Work out the finished part from the listing and answer in its coordinate system (mm). Coordinates: 2 decimals unless noted, no trailing zeros. Order: outer loops, then holes, each group sorted by start corner. A loop starts at its lowest first (then second) coordinate and runs counter-clockwise, first axis right, second up. Notation, with made-up numbers: M -34.5,11.5 L 8.5,11.5 A32 cw 8.5,49.5 Z; hole C -8.75,4.5 d3. An arc over 180 degrees is marked long. Use a Markdown table: item, result.
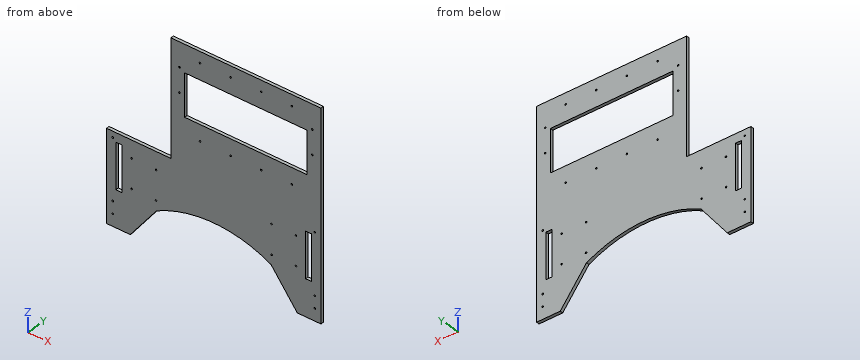
from build123d import *

# Parameters (mm, degrees)
SKETCH1_R           = 1.63195
SKETCH1_W           = 254
SKETCH1_H           = 88.9
SKETCH1_W_2         = 12.7
SKETCH1_H_2         = 95.25
BOSS_EXTRUDE1_DEPTH = 6.35
CUT_EXTRUDE1_REACH  = 621.735
SKETCH2_R           = 1.63195
CUT_EXTRUDE2_REACH  = 621.735
SKETCH4_R           = 1.63195


with BuildPart() as part:
    # Sketch1 → Boss-Extrude1 (new body)
    with BuildSketch(Plane(origin=(0, 0, 0), x_dir=(1, 0, 0), z_dir=(0, 1, 0))):
        with BuildLine():
            Line((-444.5, 431.8), (-395.456941666, 431.8))
            Line((-395.456941666, 431.8), (-340.943704665, 359.56166268))
            ThreePointArc((-340.943704665, 359.56166268), (-222.25, 330.203093028), (-103.556295335, 359.56166268))
            Line((-103.556295335, 359.56166268), (-49.043058334, 431.8))
            Line((-49.043058334, 431.8), (0, 431.8))
            Line((0, 431.8), (0, 0))
            Line((0, 0), (-311.15, 0))
            Line((-311.15, 0), (-311.15, 241.3))
            Line((-311.15, 241.3), (-444.5, 241.3))
            Line((-444.5, 241.3), (-444.5, 431.8))
        make_face()
        with Locations(Location((-250.825, 23.368, 0), (0, 0, 270))):
            Circle(SKETCH1_R, mode=Mode.SUBTRACT)
        with Locations(Location((-187.325, 23.368, 0), (0, 0, 270))):
            Circle(SKETCH1_R, mode=Mode.SUBTRACT)
        with Locations(Location((-187.325, 179.8955, 0), (0, 0, 270))):
            Circle(SKETCH1_R, mode=Mode.SUBTRACT)
        with Locations(Location((-250.825, 179.8955, 0), (0, 0, 270))):
            Circle(SKETCH1_R, mode=Mode.SUBTRACT)
        with Locations(Location((-123.825, 179.8955, 0), (0, 0, 270))):
            Circle(SKETCH1_R, mode=Mode.SUBTRACT)
        with Locations(Location((-60.325, 179.8955, 0), (0, 0, 270))):
            Circle(SKETCH1_R, mode=Mode.SUBTRACT)
        with Locations(Location((-123.825, 23.368, 0), (0, 0, 270))):
            Circle(SKETCH1_R, mode=Mode.SUBTRACT)
        with Locations(Location((-60.325, 23.368, 0), (0, 0, 270))):
            Circle(SKETCH1_R, mode=Mode.SUBTRACT)
        with Locations((-155.575, 101.63175)):
            Rectangle(SKETCH1_W, SKETCH1_H, mode=Mode.SUBTRACT)
        with Locations((-25.4, 307.975)):
            Rectangle(SKETCH1_W_2, SKETCH1_H_2, mode=Mode.SUBTRACT)
        with Locations((-419.1, 307.975)):
            Rectangle(SKETCH1_W_2, SKETCH1_H_2, mode=Mode.SUBTRACT)
    extrude(amount=BOSS_EXTRUDE1_DEPTH)

    # Sketch2 → Cut-Extrude1 (cut, up to next)
    with BuildSketch(Plane(origin=(0, 6.35, 0), x_dir=(1, 0, 0), z_dir=(0, 1, 0)), mode=Mode.PRIVATE) as cut_extrude1_sk1:
        with Locations(Location((-293.37, 101.6, 0), (0, 0, 270))):
            Circle(SKETCH2_R)
    cut_extrude1_tool1 = extrude(cut_extrude1_sk1.sketch, amount=-CUT_EXTRUDE1_REACH, mode=Mode.PRIVATE) & part.part
    # Sketch2 → Cut-Extrude1 (cut, up to next)
    with BuildSketch(Plane(origin=(0, 6.35, 0), x_dir=(1, 0, 0), z_dir=(0, 1, 0)), mode=Mode.PRIVATE) as cut_extrude1_sk2:
        with Locations(Location((-293.37, 50.8, 0), (0, 0, 270))):
            Circle(SKETCH2_R)
    cut_extrude1_tool2 = extrude(cut_extrude1_sk2.sketch, amount=-CUT_EXTRUDE1_REACH, mode=Mode.PRIVATE) & part.part
    # Sketch2 → Cut-Extrude1 (cut, up to next)
    with BuildSketch(Plane(origin=(0, 6.35, 0), x_dir=(1, 0, 0), z_dir=(0, 1, 0)), mode=Mode.PRIVATE) as cut_extrude1_sk3:
        with Locations(Location((-17.78, 101.6, 0), (0, 0, 270))):
            Circle(SKETCH2_R)
    cut_extrude1_tool3 = extrude(cut_extrude1_sk3.sketch, amount=-CUT_EXTRUDE1_REACH, mode=Mode.PRIVATE) & part.part
    # Sketch2 → Cut-Extrude1 (cut, up to next)
    with BuildSketch(Plane(origin=(0, 6.35, 0), x_dir=(1, 0, 0), z_dir=(0, 1, 0)), mode=Mode.PRIVATE) as cut_extrude1_sk4:
        with Locations(Location((-17.78, 50.8, 0), (0, 0, 270))):
            Circle(SKETCH2_R)
    cut_extrude1_tool4 = extrude(cut_extrude1_sk4.sketch, amount=-CUT_EXTRUDE1_REACH, mode=Mode.PRIVATE) & part.part
    add(cut_extrude1_tool1.solids().sort_by_distance((-293.37, 6.35, -101.6))[0], mode=Mode.SUBTRACT)
    add(cut_extrude1_tool2.solids().sort_by_distance((-293.37, 6.35, -50.8))[0], mode=Mode.SUBTRACT)
    add(cut_extrude1_tool3.solids().sort_by_distance((-17.78, 6.35, -101.6))[0], mode=Mode.SUBTRACT)
    add(cut_extrude1_tool4.solids().sort_by_distance((-17.78, 6.35, -50.8))[0], mode=Mode.SUBTRACT)

    # Sketch4 → Cut-Extrude2 (cut, up to next)
    with BuildSketch(Plane(origin=(0, 6.35, 0), x_dir=(1, 0, 0), z_dir=(0, 1, 0)), mode=Mode.PRIVATE) as cut_extrude2_sk1:
        with Locations(Location((-102.439928105, 339.392140239, 0), (0, 0, 270))):
            Circle(SKETCH4_R)
    cut_extrude2_tool1 = extrude(cut_extrude2_sk1.sketch, amount=-CUT_EXTRUDE2_REACH, mode=Mode.PRIVATE) & part.part
    # Sketch4 → Cut-Extrude2 (cut, up to next)
    with BuildSketch(Plane(origin=(0, 6.35, 0), x_dir=(1, 0, 0), z_dir=(0, 1, 0)), mode=Mode.PRIVATE) as cut_extrude2_sk2:
        with Locations(Location((-51.640295705, 339.198883781, 0), (0, 0, 270))):
            Circle(SKETCH4_R)
    cut_extrude2_tool2 = extrude(cut_extrude2_sk2.sketch, amount=-CUT_EXTRUDE2_REACH, mode=Mode.PRIVATE) & part.part
    # Sketch4 → Cut-Extrude2 (cut, up to next)
    with BuildSketch(Plane(origin=(0, 6.35, 0), x_dir=(1, 0, 0), z_dir=(0, 1, 0)), mode=Mode.PRIVATE) as cut_extrude2_sk3:
        with Locations(Location((-102.55625, 278.238883781, 0), (0, 0, 270))):
            Circle(SKETCH4_R)
    cut_extrude2_tool3 = extrude(cut_extrude2_sk3.sketch, amount=-CUT_EXTRUDE2_REACH, mode=Mode.PRIVATE) & part.part
    # Sketch4 → Cut-Extrude2 (cut, up to next)
    with BuildSketch(Plane(origin=(0, 6.35, 0), x_dir=(1, 0, 0), z_dir=(0, 1, 0)), mode=Mode.PRIVATE) as cut_extrude2_sk4:
        with Locations(Location((-51.75625, 278.238883781, 0), (0, 0, 270))):
            Circle(SKETCH4_R)
    cut_extrude2_tool4 = extrude(cut_extrude2_sk4.sketch, amount=-CUT_EXTRUDE2_REACH, mode=Mode.PRIVATE) & part.part
    # Sketch4 → Cut-Extrude2 (cut, up to next)
    with BuildSketch(Plane(origin=(0, 6.35, 0), x_dir=(1, 0, 0), z_dir=(0, 1, 0)), mode=Mode.PRIVATE) as cut_extrude2_sk5:
        with Locations(Location((-392.74375, 278.238883781, 0), (0, 0, 270))):
            Circle(SKETCH4_R)
    cut_extrude2_tool5 = extrude(cut_extrude2_sk5.sketch, amount=-CUT_EXTRUDE2_REACH, mode=Mode.PRIVATE) & part.part
    # Sketch4 → Cut-Extrude2 (cut, up to next)
    with BuildSketch(Plane(origin=(0, 6.35, 0), x_dir=(1, 0, 0), z_dir=(0, 1, 0)), mode=Mode.PRIVATE) as cut_extrude2_sk6:
        with Locations(Location((-341.94375, 278.238883781, 0), (0, 0, 270))):
            Circle(SKETCH4_R)
    cut_extrude2_tool6 = extrude(cut_extrude2_sk6.sketch, amount=-CUT_EXTRUDE2_REACH, mode=Mode.PRIVATE) & part.part
    # Sketch4 → Cut-Extrude2 (cut, up to next)
    with BuildSketch(Plane(origin=(0, 6.35, 0), x_dir=(1, 0, 0), z_dir=(0, 1, 0)), mode=Mode.PRIVATE) as cut_extrude2_sk7:
        with Locations(Location((-392.859704295, 339.198883781, 0), (0, 0, 270))):
            Circle(SKETCH4_R)
    cut_extrude2_tool7 = extrude(cut_extrude2_sk7.sketch, amount=-CUT_EXTRUDE2_REACH, mode=Mode.PRIVATE) & part.part
    # Sketch4 → Cut-Extrude2 (cut, up to next)
    with BuildSketch(Plane(origin=(0, 6.35, 0), x_dir=(1, 0, 0), z_dir=(0, 1, 0)), mode=Mode.PRIVATE) as cut_extrude2_sk8:
        with Locations(Location((-342.060071895, 339.392140239, 0), (0, 0, 270))):
            Circle(SKETCH4_R)
    cut_extrude2_tool8 = extrude(cut_extrude2_sk8.sketch, amount=-CUT_EXTRUDE2_REACH, mode=Mode.PRIVATE) & part.part
    # Sketch4 → Cut-Extrude2 (cut, up to next)
    with BuildSketch(Plane(origin=(0, 6.35, 0), x_dir=(1, 0, 0), z_dir=(0, 1, 0)), mode=Mode.PRIVATE) as cut_extrude2_sk9:
        with Locations(Location((-12.7, 406.4, 0), (0, 0, 270))):
            Circle(SKETCH4_R)
    cut_extrude2_tool9 = extrude(cut_extrude2_sk9.sketch, amount=-CUT_EXTRUDE2_REACH, mode=Mode.PRIVATE) & part.part
    # Sketch4 → Cut-Extrude2 (cut, up to next)
    with BuildSketch(Plane(origin=(0, 6.35, 0), x_dir=(1, 0, 0), z_dir=(0, 1, 0)), mode=Mode.PRIVATE) as cut_extrude2_sk10:
        with Locations(Location((-12.7, 381, 0), (0, 0, 270))):
            Circle(SKETCH4_R)
    cut_extrude2_tool10 = extrude(cut_extrude2_sk10.sketch, amount=-CUT_EXTRUDE2_REACH, mode=Mode.PRIVATE) & part.part
    # Sketch4 → Cut-Extrude2 (cut, up to next)
    with BuildSketch(Plane(origin=(0, 6.35, 0), x_dir=(1, 0, 0), z_dir=(0, 1, 0)), mode=Mode.PRIVATE) as cut_extrude2_sk11:
        with Locations(Location((-12.7, 254, 0), (0, 0, 270))):
            Circle(SKETCH4_R)
    cut_extrude2_tool11 = extrude(cut_extrude2_sk11.sketch, amount=-CUT_EXTRUDE2_REACH, mode=Mode.PRIVATE) & part.part
    # Sketch4 → Cut-Extrude2 (cut, up to next)
    with BuildSketch(Plane(origin=(0, 6.35, 0), x_dir=(1, 0, 0), z_dir=(0, 1, 0)), mode=Mode.PRIVATE) as cut_extrude2_sk12:
        with Locations(Location((-431.8, 254, 0), (0, 0, 270))):
            Circle(SKETCH4_R)
    cut_extrude2_tool12 = extrude(cut_extrude2_sk12.sketch, amount=-CUT_EXTRUDE2_REACH, mode=Mode.PRIVATE) & part.part
    # Sketch4 → Cut-Extrude2 (cut, up to next)
    with BuildSketch(Plane(origin=(0, 6.35, 0), x_dir=(1, 0, 0), z_dir=(0, 1, 0)), mode=Mode.PRIVATE) as cut_extrude2_sk13:
        with Locations(Location((-431.8, 381, 0), (0, 0, 270))):
            Circle(SKETCH4_R)
    cut_extrude2_tool13 = extrude(cut_extrude2_sk13.sketch, amount=-CUT_EXTRUDE2_REACH, mode=Mode.PRIVATE) & part.part
    # Sketch4 → Cut-Extrude2 (cut, up to next)
    with BuildSketch(Plane(origin=(0, 6.35, 0), x_dir=(1, 0, 0), z_dir=(0, 1, 0)), mode=Mode.PRIVATE) as cut_extrude2_sk14:
        with Locations(Location((-431.8, 406.4, 0), (0, 0, 270))):
            Circle(SKETCH4_R)
    cut_extrude2_tool14 = extrude(cut_extrude2_sk14.sketch, amount=-CUT_EXTRUDE2_REACH, mode=Mode.PRIVATE) & part.part
    add(cut_extrude2_tool1.solids().sort_by_distance((-102.439928, 6.35, -339.39214))[0], mode=Mode.SUBTRACT)
    add(cut_extrude2_tool2.solids().sort_by_distance((-51.640296, 6.35, -339.198884))[0], mode=Mode.SUBTRACT)
    add(cut_extrude2_tool3.solids().sort_by_distance((-102.55625, 6.35, -278.238884))[0], mode=Mode.SUBTRACT)
    add(cut_extrude2_tool4.solids().sort_by_distance((-51.75625, 6.35, -278.238884))[0], mode=Mode.SUBTRACT)
    add(cut_extrude2_tool5.solids().sort_by_distance((-392.74375, 6.35, -278.238884))[0], mode=Mode.SUBTRACT)
    add(cut_extrude2_tool6.solids().sort_by_distance((-341.94375, 6.35, -278.238884))[0], mode=Mode.SUBTRACT)
    add(cut_extrude2_tool7.solids().sort_by_distance((-392.859704, 6.35, -339.198884))[0], mode=Mode.SUBTRACT)
    add(cut_extrude2_tool8.solids().sort_by_distance((-342.060072, 6.35, -339.39214))[0], mode=Mode.SUBTRACT)
    add(cut_extrude2_tool9.solids().sort_by_distance((-12.7, 6.35, -406.4))[0], mode=Mode.SUBTRACT)
    add(cut_extrude2_tool10.solids().sort_by_distance((-12.7, 6.35, -381))[0], mode=Mode.SUBTRACT)
    add(cut_extrude2_tool11.solids().sort_by_distance((-12.7, 6.35, -254))[0], mode=Mode.SUBTRACT)
    add(cut_extrude2_tool12.solids().sort_by_distance((-431.8, 6.35, -254))[0], mode=Mode.SUBTRACT)
    add(cut_extrude2_tool13.solids().sort_by_distance((-431.8, 6.35, -381))[0], mode=Mode.SUBTRACT)
    add(cut_extrude2_tool14.solids().sort_by_distance((-431.8, 6.35, -406.4))[0], mode=Mode.SUBTRACT)


solid = part.part
1. Section A-A on z = -267 is taken. Determine the outline of the cut face in (x, y), then the cut area to 3 significant figures.
Answers below:
| item | result |
|---|---|
| outline | M -444.5,0 L -425.45,0 L -425.45,6.35 L -444.5,6.35 Z; M -412.75,0 L -31.75,0 L -31.75,6.35 L -412.75,6.35 Z; M -19.05,0 L 0,0 L 0,6.35 L -19.05,6.35 Z |
| area | 2,660 mm² |
2. Section D-D on y = 4.5 is taken. Give the number of separate pieces and of enclosed holes in the cut face, then the cut area to 3 significant figures.
Answers below:
| item | result |
|---|---|
| separate pieces | 1 |
| enclosed holes | 29 |
| area | 109,000 mm² |
3. Flat-ended cylindrical pins translate along their axes: P1, Ø1.9, axis at y = 4, z = -107, coming from the -X side; P2, Ø3, axis at x = -312.5, y = 3.5, coming from the -Z side; P3, Ø1.9, axis at x = -407.5, y = 3, coming from the +Z side. Find the tip coordinate at first contact, or state that the pin passes through.
Answers below:
| item | result |
|---|---|
| P1 | x = -311.15 |
| P2 | z = -347.31 |
| P3 | z = -241.3 |
4. Find the intervals of material crossed by probe 1 along X at (y, z) = (3.25, -254); probe 2 along X at (y, z) = (4.5, -101.6) (3 decimals); probe 3 along X at (y, z) = (4, -112) (3 decimals), in increasing order.
Answers below:
| item | result |
|---|---|
| probe 1 | -444.5 to -433.43, -430.17 to -14.33, -11.07 to 0 |
| probe 2 | -311.15 to -295.002, -291.738 to -282.575, -28.575 to -19.412, -16.148 to 0 |
| probe 3 | -311.15 to -282.575, -28.575 to 0 |
5. Section C-C on z = -93 is taken. Determine the outline of the cut face in (x, y) (3 decimals), then the cut area to 3 significant figures.
Answers below:
| item | result |
|---|---|
| outline | M -311.15,0 L -282.575,0 L -282.575,6.35 L -311.15,6.35 Z; M -28.575,0 L 0,0 L 0,6.35 L -28.575,6.35 Z |
| area | 363 mm² |
6. Section B-B on x = -272 is taken. Determine the outline of the cut face in (y, z).
Answers below:
| item | result |
|---|---|
| outline | M 0,-335.11 L 6.35,-335.11 L 6.35,-146.08 L 0,-146.08 Z; M 0,-57.18 L 6.35,-57.18 L 6.35,0 L 0,0 Z |
